Design review of the part built by this model. Coordinates are the model's own, in mm. Face numbers are marked on the shaded views. A direction names the side the tool comes from. Give positions to 0.01 mm unless a question says otherwise; leave off trailing zeros. Write each loop counter-clockwise with the first axis right and the second up, starting at its lowest first coordinate (ties: lowest second). Pieces come first, ordered by that corner, then holes. Notation, with made-up numbers: (-6, -39) -> (42, -39) arc R18 ccw to (42, -15) -> close; hole circle Ø1 at (-25, 34). An arc over 180 degrees is marked (long way). Answer as a JSON object with one key per item and string values.
```python
from build123d import *

# Parameters (mm, degrees)
CROQUIS1_R              = 7
CROQUIS1_R_2            = 4.85
SALIENTE_EXTRUIR1_DEPTH = 3.5
CROQUIS4_W              = 8.235883517
CROQUIS4_H              = 32.578937154
CORTAR_EXTRUIR4_DEPTH   = 4
CROQUIS5_R              = 7
CROQUIS5_R_2            = 4
SALIENTE_EXTRUIR2_DEPTH = 2
SALIENTE_EXTRUIR3_START = 2
CROQUIS6_R              = 7
CROQUIS6_R_2            = 4
SALIENTE_EXTRUIR3_DEPTH = 2


with BuildPart() as part:
    # Croquis1 → Saliente-Extruir1 (new body)
    # profile 1 of 3: a face of its own
    with BuildSketch(Plane.XY):
        with BuildLine():
            ThreePointArc((-4.949747468, -4.949747468), (-4.949747468, 4.949747468), (4.949747468, 4.949747468))
            Line((4.949747468, 4.949747468), (1, 8.899494937))
            Line((1, 8.899494937), (1, 21.100505063))
            Line((1, 21.100505063), (4.949747468, 25.050252532))
            ThreePointArc((4.949747468, 25.050252532), (-4.949747468, 25.050252532), (-4.949747468, 34.949747468))
            Line((-4.949747468, 34.949747468), (-13, 26.899494937))
            Line((-13, 26.899494937), (-13, 3.100505063))
            Line((-13, 3.100505063), (-4.949747468, -4.949747468))
        make_face()
    # profile 2 of 3: a face of its own
    with BuildSketch(Plane.XY):
        with Locations((0, 30)):
            Circle(CROQUIS1_R)
        with Locations((0, 30)):
            Circle(CROQUIS1_R_2, mode=Mode.SUBTRACT)
    # profile 3 of 3: a face of its own
    with BuildSketch(Plane.XY):
        Circle(CROQUIS1_R)
        Circle(CROQUIS1_R_2, mode=Mode.SUBTRACT)
    extrude(amount=SALIENTE_EXTRUIR1_DEPTH)

    # Croquis4 → Cortar-Extruir4 (cut)
    with BuildSketch(Plane.XY.offset(3.5)):
        with Locations((-14.117941759, 13.61002636)):
            Rectangle(CROQUIS4_W, CROQUIS4_H)
    extrude(amount=-CORTAR_EXTRUIR4_DEPTH, mode=Mode.SUBTRACT)

    # Croquis5 → Saliente-Extruir2 (add)
    with BuildSketch(Plane.XY.offset(3.5)):
        with Locations(Location((0, 0, 0), (0, 0, 225))):
            Circle(CROQUIS5_R)
        Circle(CROQUIS5_R_2, mode=Mode.SUBTRACT)
    extrude(amount=SALIENTE_EXTRUIR2_DEPTH)

    # Croquis6 → Saliente-Extruir3 (add)
    with BuildSketch(Plane(origin=(0, 0, 0), x_dir=(-1, 0, 0), z_dir=(0, 0, -1)).offset(SALIENTE_EXTRUIR3_START)):
        with Locations((0, 30)):
            Circle(CROQUIS6_R)
        with Locations((0, 30)):
            Circle(CROQUIS6_R_2, mode=Mode.SUBTRACT)
    extrude(amount=-SALIENTE_EXTRUIR3_DEPTH)


solid = part.part
```
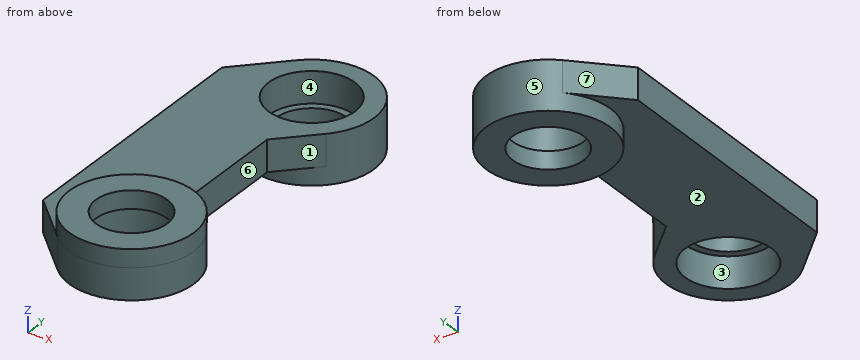
(1) We need section B-B, the plane z = 1.75. State the section outline as (x, y) points.
Here are the results:
{"outline": "(-10, 0.1) -> (-4.95, -4.95) arc R7 ccw to (4.95, 4.95) -> (1, 8.9) -> (1, 21.1) -> (4.95, 25.05) arc R7 ccw to (-4.95, 34.95) -> (-10, 29.9) -> close; hole circle Ø9.7 at (0, 0); hole circle Ø9.7 at (0, 30)"}
(2) For line 1 along Y through (x, z) = (0, 1.1); line 2 along Y through (x, z) = (0, -0.65); line 3 along Z through (x, y) = (4.75, 2), list the stretches that pass through material, from the lowest coordinate up.
Here are the results:
{"line 1": "y = -7 to -4.85, 4.85 to 25.15, 34.85 to 37", "line 2": "y = 23 to 26, 34 to 37", "line 3": "z = 0 to 5.5"}
(3) For the marked faces 4, 5, 6 and 7, list the 3-axis set-ups (+Z, -Z, +X, -X, +Y, -Y) from which the entire face can be reached by the end or side of a thin tool; tool diameter is ignored.
Here are the results:
{"face 4": "+Z", "face 5": "-Z", "face 6": "+Z, -Z, +X", "face 7": "+Z, -Z, -X, +Y"}
(4) We need section D-D, the plane x = 6. State the section outline as (y, z) points.
Here are the results:
{"outline": "(-3.61, 0) -> (3.61, 0) -> (3.61, 5.5) -> (-3.61, 5.5) -> close; (26.39, -2) -> (33.61, -2) -> (33.61, 3.5) -> (26.39, 3.5) -> close"}
(5) We need section A-A, the plane x = 0. State the section outline as (y, z) points.
Here are the results:
{"outline": "(-7, 0) -> (-4.85, 0) -> (-4.85, 3.5) -> (-4, 3.5) -> (-4, 5.5) -> (-7, 5.5) -> close; (4, 3.5) -> (4.85, 3.5) -> (4.85, 0) -> (23, 0) -> (23, -2) -> (26, -2) -> (26, 0) -> (25.15, 0) -> (25.15, 3.5) -> (7, 3.5) -> (7, 5.5) -> (4, 5.5) -> close; (34, -2) -> (37, -2) -> (37, 3.5) -> (34.85, 3.5) -> (34.85, 0) -> (34, 0) -> close"}
(6) We need section C-C, the plane y = 28. State the section outline as (x, z) points.
Here are the results:
{"outline": "(-10, 0) -> (-6.71, 0) -> (-6.71, -2) -> (-3.46, -2) -> (-3.46, 0) -> (-4.42, 0) -> (-4.42, 3.5) -> (-10, 3.5) -> close; (3.46, -2) -> (6.71, -2) -> (6.71, 3.5) -> (4.42, 3.5) -> (4.42, 0) -> (3.46, 0) -> close"}
(7) The part is to be moulded in two halves that separate along X. For the marked faces 1, 2 and 3, say which applies: +X half, -X half, draft (parallel to the pull), parting line (faces both ways), or undercut.
Here are the results:
{"face 1": "+X half", "face 2": "draft", "face 3": "undercut"}
(8) Clearance check with flat-ended pins moving along their axes: pin 1 (4 mm diameter, centred on x = 4.5, z = 3, fed in from +Y); pin 2 (2 mm diameter, centred on x = -5.5, y = 29, fed in from +Z); pin 3 (1 mm diameter, centred on x = -8, y = 8.5, fed in from -Z); pin 4 (4 mm diameter, centred on x = -0.5, z = 1.5, fed in from -Y). State where each tip first meets the part, or that it passes through.
Here are the results:
{"pin 1": "stops at y = 36.54", "pin 2": "stops at z = 3.5", "pin 3": "stops at z = 0", "pin 4": "stops at y = -7"}
